Drawing for the job (mm, zero at the part's lowest x, y, z). A direction names the side the tool comes from. Coordinates: 2 decimals unless noted, no trailing zeros. Write each loop counter-clockwise with the first axis right and the second up, starting at its lowest first coordinate (ties: lowest second). Pieces come first, ordered by that corner, then holes. Notation, with made-up numbers: (65.5, 61) -> (83.5, 61) arc R16 ccw to (83.5, 66) -> close; hole circle Ø8 at (-4.75, 60.5). An arc over 180 degrees is marked (long way). Write each question's results on one line, items separated by ' | '. Start each with the question number.
Q1. Drill centre lines: line 1 (Y direction, x = 17.5, z = 2.25); line 2 (X direction, y = 12.5, z = 2.75); line 3 (Y direction, x = 13, z = 4.3) (1 decimal). Where is each one in solid material? Low to high.
Q2. Saw through at C-C on y = 16. Give the cut face in (x, z).
Q3. Drop flat-ended pins along their axis: pin 1 Ø4.5 at (x, y) = (16, 4) entering from +Z; pin 2 Ø1.5 at (x, z) = (17, 2) entering from -Y; pin 3 Ø2 at (y, z) = (28, 3) entering from +X; pin 4 Ø1 at (x, z) = (9, 3) entering from -Y. Give the stop position or say it passes through.
Q4. Tool access for the marked faces 4, 5 and 6: list every direction of +Z, -Z, +X, -X, +Y, -Y with a clear straight run to the whole face (end or side of a thin tool).
Q5. Two-plate mould, pull along X, no slides. Class the marked faces 1, 2 and 3: released by +X, released by -X, zero draft, split by the parting line, or undercut.
Q6. Saw through at A-A on y = 22. Count the separate pieces of the cut face and the enclosed holes in it, and give its area (3 significant figures).
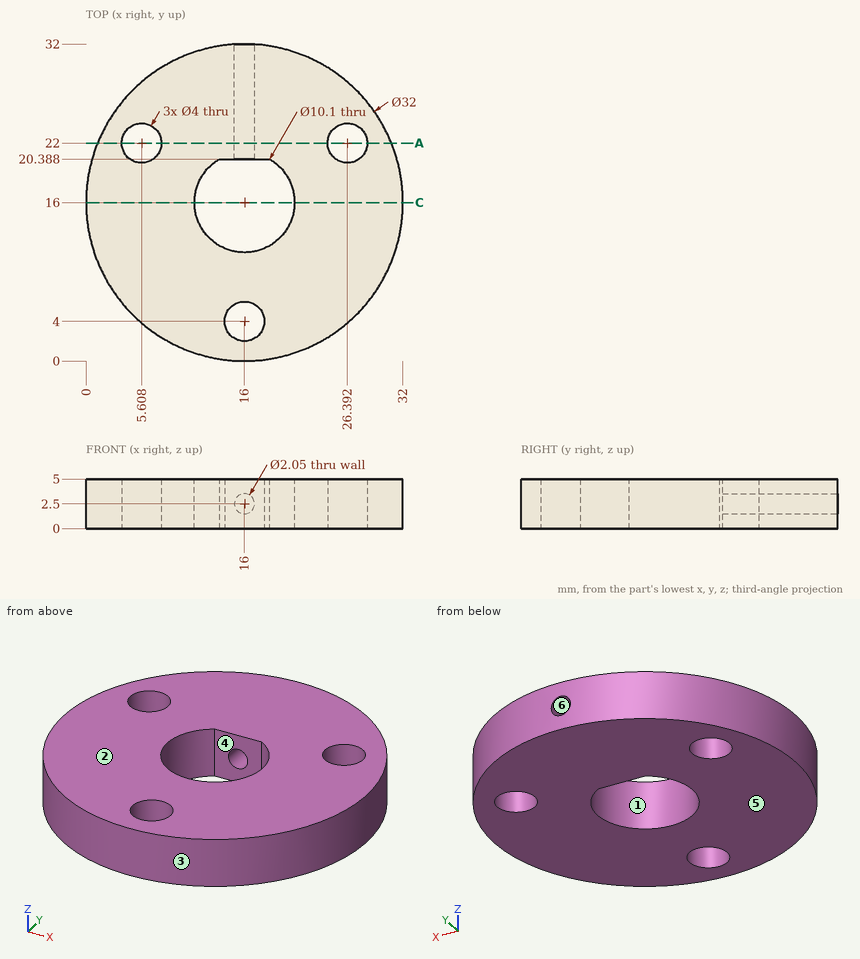
Returned:
1) line 1: y = 0.07 to 2.68, 5.32 to 11.18, 20.39 to 31.93 | line 2: x = 0.39 to 12.36, 19.64 to 31.61 | line 3: y = 0.3 to 11.9, 20.1 to 31.7
2) outline: (0, 0) -> (10.95, 0) -> (10.95, 5) -> (0, 5) -> close; (21.05, 0) -> (32, 0) -> (32, 5) -> (21.05, 5) -> close
3) pin 1: stops at z = 5 | pin 2: stops at y = 0 | pin 3: stops at x = 27.62 | pin 4: stops at y = 1.38
4) face 4: +Z, -Z | face 5: -Z, +X, -X, +Y, -Y | face 6: +Y
5) face 1: undercut | face 2: zero draft | face 3: split by the parting line
6) separate pieces: 3 | enclosed holes: 1 | area: 105 mm2
